Verification items for the finished model (mm, model axes). A direction names the side the tool comes from. Coordinates: 2 decimals unless noted, no trailing zeros. Order: outer loops, then holes, each group sorted by start corner. A loop starts at its lowest first (then second) coordinate and runs counter-clockwise, first axis right, second up. Notation, with made-up numbers: (-26.75, 44) -> (-17.75, 44) arc R21 cw to (-17.75, 82) -> close; hole circle Ø2 at (-7.5, 86). An arc over 180 degrees is marked (long way). Use CSV: the item, a comma, the result in double quotes. Start each with the question number.
1) Tool access check on faces 1 (the cylindrical face through (14.1, 0, 2.1)), 2 (the cylindrical face through (17.75, -0.03, 1.14)), 3 (the cylindrical face through (-17.75, -0.17, 1.14)), 4 (the flat face through (15.5, 0, 2)). Record the directions out of +Z, -Z, +X, -X, +Y, -Y that give a thin tool (end or side, any length) a straight path to the whole face; none if there is none.
2) Scan lines: line 1 along X through (y, z) = (-0.6, 0.8); line 2 along X through (y, z) = (-1.55, 2.45); line 3 along Z through (x, y) = (1.5, -1.75). Record each from-to range of solid material in increasing order.
3) Sectioned sample at C-C on x = 11.5. Record the boundary of the cut face in (y, z).
4) Go/stop test with flat-tipped pins: pin 1 (1 mm diameter, centred on y = -1, z = 2.5, fed in from -X); pin 2 (1.7 mm diameter, centred on y = 0, z = 1.5, fed in from +X). Record where each tip stops, or that it passes through.
5) Release check for a two-part mould opening along Z. For faces 5 (the cylindrical face through (-17.9, -0.2, 2.1)), 6 (the cylindrical face through (-14.25, -0.23, 1.14)), 7 (the conical face through (17.2, 0, 3.1)) record: released by +Z, released by -Z, zero draft, split by the parting line, or undercut.
6) Sectioned sample at B-B on x = -4.5. Record the boundary of the cut face in (y, z).
7) Sectioned sample at A-A on z = 1. Record the boundary of the cut face in (x, y).
8) Sectioned sample at D-D on z = 2.9. Record the boundary of the cut face in (x, y).
from build123d import *

# Parameters (mm, degrees)
SKICA2_W                 = 50
SKICA2_H                 = 4.2
SKICA2_W_2               = 18
SKICA2_H_2               = 1
P_IDAT_VYSUNUT_M2_DEPTH  = 0.4
SKICA3_R                 = 1.75
P_IDAT_VYSUNUT_M3_DEPTH  = 1.5
SKICA5_R                 = 1.9
P_IDAT_VYSUNUT_M5_DEPTH  = 2
ZKOSEN_2_SIZE            = 1.5
SKICA7_W                 = 1
SKICA7_H                 = 5
ODEBRAT_VYSUNUT_M1_DEPTH = 3.5


with BuildPart() as part:
    # Skica2 → Přidat vysunutím2 (new body)
    with BuildSketch(Plane.XY):
        Rectangle(SKICA2_W, SKICA2_H)
        with Locations((0, -0.2)):
            Rectangle(SKICA2_W_2, SKICA2_H_2, mode=Mode.SUBTRACT)
    extrude(amount=P_IDAT_VYSUNUT_M2_DEPTH)

    # Skica3 → Přidat vysunutím3 (add)
    with BuildSketch(Plane.XY.offset(0.4)):
        with Locations((-16, -0.2)):
            Circle(SKICA3_R)
        with Locations((16, 0)):
            Circle(SKICA3_R)
    extrude(amount=P_IDAT_VYSUNUT_M3_DEPTH)

    # Skica5 → Přidat vysunutím5 (add)
    with BuildSketch(Plane.XY.offset(1.9)):
        with Locations((-16, -0.2)):
            Circle(SKICA5_R)
        with Locations((16, 0)):
            Circle(SKICA5_R)
    extrude(amount=P_IDAT_VYSUNUT_M5_DEPTH)

    # Zkosení2
    zkosen_2_edges = [part.edges().sort_by_distance(p)[0] for p in [
        (-17.9, -0.2, 3.9),
        (14.1, 0, 3.9),
    ]]
    chamfer(zkosen_2_edges, length=ZKOSEN_2_SIZE)

    # Skica7 → Odebrat vysunutím1 (cut)
    with BuildSketch(Plane.XY.offset(3.9)):
        with Locations((-16, -0.2)):
            Rectangle(SKICA7_W, SKICA7_H)
        with Locations((16, 0)):
            Rectangle(SKICA7_W, SKICA7_H)
    extrude(amount=-ODEBRAT_VYSUNUT_M1_DEPTH, mode=Mode.SUBTRACT)


solid = part.part
Answers follow:
1,face 1,"+Z"
1,face 2,"+X"
1,face 3,"-X"
1,face 4,"+Z, +Y, -Y"
2,line 1,"x = -17.7 to -16.5, -15.5 to -14.3, 14.36 to 15.5, 16.5 to 17.64"
2,line 2,"x = -17.26 to -16.5, -15.5 to -14.74, 14.99 to 15.5, 16.5 to 17.01"
2,line 3,"z = 0 to 0.4"
3,outline,"(-2.1, 0) -> (2.1, 0) -> (2.1, 0.4) -> (-2.1, 0.4) -> close"
4,pin 1,"stops at x = -17.87"
4,pin 2,"stops at x = 17.9"
5,face 5,"zero draft"
5,face 6,"undercut"
5,face 7,"released by +Z"
6,outline,"(-2.1, 0) -> (-0.7, 0) -> (-0.7, 0.4) -> (-2.1, 0.4) -> close; (0.3, 0) -> (2.1, 0) -> (2.1, 0.4) -> (0.3, 0.4) -> close"
7,outline,"(-16.5, -1.88) -> (-16.5, 1.48) arc R1.75 ccw to start; (-15.5, -1.88) arc R1.75 ccw to (-15.5, 1.48) -> close; (15.5, -1.68) -> (15.5, 1.68) arc R1.75 ccw to start; (16.5, -1.68) arc R1.75 ccw to (16.5, 1.68) -> close"
8,outline,"(-16.5, -1.51) -> (-16.5, 1.11) arc R1.4 ccw to start; (-15.5, -1.51) arc R1.4 ccw to (-15.5, 1.11) -> close; (15.5, -1.31) -> (15.5, 1.31) arc R1.4 ccw to start; (16.5, -1.31) arc R1.4 ccw to (16.5, 1.31) -> close"
